```python
from build123d import *

# Parameters (mm, degrees)
BOSS_EXTRUDE5_DEPTH      = 10
BOSS_EXTRUDE5_DEPTH_BACK = 10
BOSS_EXTRUDE6_DEPTH      = 25
BOSS_EXTRUDE6_DEPTH_BACK = 10
SKETCH1_8_W              = 5
SKETCH1_8_H              = 15
BOSS_EXTRUDE7_START      = 20
SKETCH1_9_W              = 4
SKETCH1_9_H              = 15
BOSS_EXTRUDE7_DEPTH      = 5
BOSS_EXTRUDE8_DEPTH      = 10
BOSS_EXTRUDE8_DEPTH_BACK = 10
BOSS_EXTRUDE9_DEPTH      = 10
BOSS_EXTRUDE9_DEPTH_BACK = 10
SKETCH1_11_W             = 36
SKETCH1_11_H             = 3
CUT_EXTRUDE2_DEPTH       = 70.846371595
CUT_EXTRUDE2_DEPTH_BACK  = 70.846371595
SKETCH2_R                = 2.5


with BuildPart() as part:
    # Sketch1 → Boss-Extrude5 (new, two sides: drawn at the far end of the back side and taken through both)
    with BuildSketch(Plane(origin=(0, 0, 0), x_dir=(0, 0, -1), z_dir=(1, 0, 0)).offset(-BOSS_EXTRUDE5_DEPTH_BACK)):
        Polygon((-7, 41.875), (-7, 7.5), (-2, 7.5), (-2, 36.875), (2, 36.875), (2, 7.5), (7, 7.5), (7, 41.875), align=None)
    extrude(amount=BOSS_EXTRUDE5_DEPTH + BOSS_EXTRUDE5_DEPTH_BACK)

    # Sketch1_8 → Boss-Extrude6 (add, two sides: drawn at the far end of the back side and taken through both)
    with BuildSketch(Plane(origin=(0, 0, 0), x_dir=(0, 0, -1), z_dir=(1, 0, 0)).offset(-BOSS_EXTRUDE6_DEPTH_BACK)):
        with Locations((-4.5, 0)):
            Rectangle(SKETCH1_8_W, SKETCH1_8_H)
        with Locations((4.5, 0)):
            Rectangle(SKETCH1_8_W, SKETCH1_8_H)
    extrude(amount=BOSS_EXTRUDE6_DEPTH + BOSS_EXTRUDE6_DEPTH_BACK)

    # Sketch1_9 → Boss-Extrude7 (add)
    with BuildSketch(Plane(origin=(0, 0, 0), x_dir=(0, 0, -1), z_dir=(1, 0, 0)).offset(BOSS_EXTRUDE7_START)):
        Rectangle(SKETCH1_9_W, SKETCH1_9_H)
    extrude(amount=BOSS_EXTRUDE7_DEPTH)

    # Sketch1_10 → Boss-Extrude8 (add, two sides: drawn at the far end of the back side and taken through both)
    with BuildSketch(Plane(origin=(0, 0, 0), x_dir=(0, 0, -1), z_dir=(1, 0, 0)).offset(-BOSS_EXTRUDE8_DEPTH_BACK)):
        Polygon((-2, -7.5), (-7, -7.5), (-7, -10.125), (-7, -13.125), (-7, -41.875), (7, -41.875), (7, -13.125), (7, -10.125), (7, -7.5), (2, -7.5), (2, -36.875), (-2, -36.875), align=None)
    extrude(amount=BOSS_EXTRUDE8_DEPTH + BOSS_EXTRUDE8_DEPTH_BACK)

    # Sketch1_11 → Boss-Extrude9 (add, two sides: drawn at the far end of the back side and taken through both)
    with BuildSketch(Plane(origin=(0, 0, 0), x_dir=(0, 0, -1), z_dir=(1, 0, 0)).offset(-BOSS_EXTRUDE9_DEPTH_BACK)):
        with Locations((25, -11.625)):
            Rectangle(SKETCH1_11_W, SKETCH1_11_H)
        with Locations((-25, -11.625)):
            Rectangle(SKETCH1_11_W, SKETCH1_11_H)
    extrude(amount=BOSS_EXTRUDE9_DEPTH + BOSS_EXTRUDE9_DEPTH_BACK)

    # Sketch2 → Cut-Extrude2 (cut, two sides: drawn at the far end of the back side and taken through both)
    with BuildSketch(Plane.XY.offset(7).offset(-CUT_EXTRUDE2_DEPTH_BACK)):
        with Locations(Location((0, 28.875, 0), (0, 0, 270))):
            Circle(SKETCH2_R)
        with Locations(Location((0, -28.875, 0), (0, 0, 90))):
            Circle(SKETCH2_R)
        with BuildLine():
            Line((0, 2.5), (12, 2.5))
            ThreePointArc((12, 2.5), (14.5, 0), (12, -2.5))
            Line((12, -2.5), (0, -2.5))
            ThreePointArc((0, -2.5), (-2.5, 0), (0, 2.5))
        make_face()
    extrude(amount=CUT_EXTRUDE2_DEPTH + CUT_EXTRUDE2_DEPTH_BACK, mode=Mode.SUBTRACT)


solid = part.part
```
Build history of the part. All positions in model axes, mm. A direction names the side the tool comes from. Round coordinates to 2 decimals unless told otherwise and drop trailing zeros. Write each loop counter-clockwise with the first axis right and the second up, starting at its lowest first coordinate (ties: lowest second). Pieces come first, ordered by that corner, then holes. Notation, with made-up numbers: (75, 56.25) - (134, 56.25) arc R14 ccw to (134, 81.25) - close; hole circle Ø9 at (-32.75, 70). An arc over 180 degrees is marked (long way). Write each question's results on one line, items separated by ' | '. Start each with the question number.
Item 1: Saw through at A-A (y = -12). Write the cut outline in (x, z).
Item 2: Wall check: L1, parallel to Z at x = 15, y = -7; L2, parallel to Y at x = 7, z = -5 (3 decimals); L3, parallel to X at y = -14.5, z = 6. Give the ranges that are in metal, low to high. Write a range as [from, to].
Item 3: Which spindle directions (+Z, -Z, +X, -X, +Y, -Y) get a long thin tool onto all of the face, cutting with end or side? Do faces 5 (the face through (-2.4, -27.7, -7)), 6 (the face through (-2.5, -0.1, -4.5)), 7 (the face through (10, 25, -3)). Say none if no direction does.
Item 4: Saw through at C-C (z = 4). Write the cut outline in (x, y) (3 decimals).
Item 5: Saw through at D-D (x = -4.5). Write the cut outline in (y, z) (3 decimals).
Item 6: Drop flat-ended pins along their axis: P1, Ø10.5, axis at x = 0, y = 14, coming from the +Z side; P2, Ø10, axis at x = 4, z = 21.5, coming from the -Y side (3 decimals); P3, Ø15.5, axis at y = 17, z = -1.5, coming from the +X side. Give the stop position or say it passes through.
Item 7: Mould opens along X. For faces 1 (the face through (20, 0, 0)), 2 (the face through (6, 2.5, 4)), 3 (the face through (-5, 1, -2)), 4 (the face through (25, 0, 0)) say: pulls with the +X half, pulls with the -X half, needs draft (parallel to the pull), parting line crosses it, or undercut.
Item 8: Saw through at B-B (y = 0). Write the cut outline in (x, z), and give its area (3 significant figures).
Results are:
1) outline: (-10, -43) - (10, -43) - (10, -2) - (-10, -2) - close; (-10, 2) - (10, 2) - (10, 43) - (-10, 43) - close
2) L1: z = [-7, -2], [2, 7] | L2: y = [-41.875, -2.5], [2.5, 41.875] | L3: x = [-10, 10]
3) face 5: -Z, +X, -X, -Y | face 6: +Z, -Z | face 7: +Z, -Z, +X, +Y
4) outline: (-10, -41.875) - (10, -41.875) - (10, -7.5) - (25, -7.5) - (25, 7.5) - (10, 7.5) - (10, 41.875) - (-10, 41.875) - close; hole circle Ø5 at (0, -28.875); hole circle Ø5 at (0, 28.875); hole (0, -2.5) - (12, -2.5) arc R2.5 ccw to (12, 2.5) - (0, 2.5) arc R2.5 ccw to start
5) outline: (-41.875, -7) - (-13.125, -7) - (-13.125, -43) - (-10.125, -43) - (-10.125, -7) - (41.875, -7) - (41.875, 7) - (-10.125, 7) - (-10.125, 43) - (-13.125, 43) - (-13.125, 7) - (-41.875, 7) - close; hole (-36.875, -2) - (36.875, -2) - (36.875, 2) - (-36.875, 2) - close
6) P1: stops at z = 7 | P2: stops at y = -13.125 | P3: stops at x = 10
7) face 1: pulls with the -X half | face 2: undercut | face 3: needs draft | face 4: pulls with the +X half
8) outline: (-10, -7) - (-2.5, -7) - (-2.5, -2) - (-10, -2) - close; (-10, 2) - (-2.5, 2) - (-2.5, 7) - (-10, 7) - close; (14.5, -7) - (25, -7) - (25, 7) - (14.5, 7) - (14.5, 2) - (20, 2) - (20, -2) - (14.5, -2) - close | area: 200 mm²
